```python
from build123d import *

# Parameters (mm, degrees)
SKETCH_1_W          = 15
SKETCH_1_H          = 5
EXTRUDE_1_DEPTH     = 10
SKETCH_2_W          = 15
SKETCH_2_H          = 15
EXTRUDE_2_DEPTH     = 5
SKETCH_3_R          = 1.25
CUT_EXTRUDE_1_DEPTH = 6
SKETCH_4_R          = 1.25
CUT_EXTRUDE_2_DEPTH = 5


with BuildPart() as part:
    # 草图1 → 凸台-拉伸1 (new body)
    with BuildSketch(Plane(origin=(0, 0, 0), x_dir=(1, 0, 0), z_dir=(0, 1, 0))):
        with Locations((7.5, 2.5)):
            Rectangle(SKETCH_1_W, SKETCH_1_H)
    extrude(amount=EXTRUDE_1_DEPTH)

    # 草图2 → 凸台-拉伸2 (add)
    with BuildSketch(Plane(origin=(0, 10, 0), x_dir=(1, 0, 0), z_dir=(0, 1, 0))):
        with Locations((7.5, -2.5)):
            Rectangle(SKETCH_2_W, SKETCH_2_H)
    extrude(amount=EXTRUDE_2_DEPTH)

    # 草图3 → 切除-拉伸1 (cut, through all)
    with BuildSketch(Plane.XY):
        with Locations((7.5, 5)):
            Circle(SKETCH_3_R)
    extrude(amount=-CUT_EXTRUDE_1_DEPTH, mode=Mode.SUBTRACT)

    # 草图4 → 切除-拉伸2 (cut)
    with BuildSketch(Plane(origin=(0, 15, 0), x_dir=(1, 0, 0), z_dir=(0, 1, 0))):
        with Locations((3, -5)):
            Circle(SKETCH_4_R)
        with Locations((12, -5)):
            Circle(SKETCH_4_R)
    extrude(amount=-CUT_EXTRUDE_2_DEPTH, mode=Mode.SUBTRACT)


solid = part.part
```
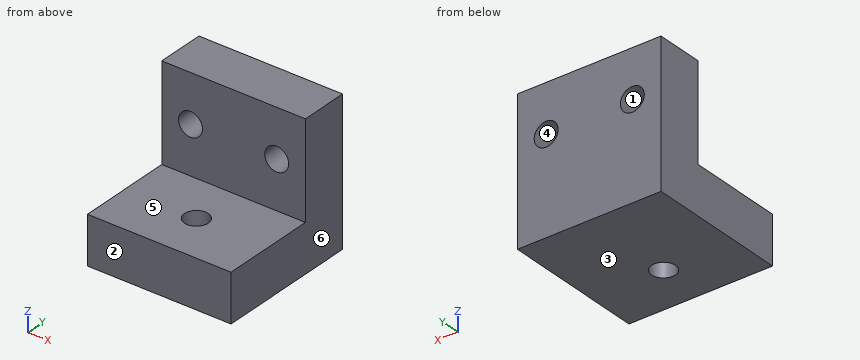
Model file for the job. Use its own axes, mm. Face numbers are marked on the shaded views. A direction names the side the tool comes from. Coordinates: 2 decimals unless noted, no trailing zeros. Write each loop counter-clockwise with the first axis right and the second up, starting at its lowest first coordinate (ties: lowest second). Pieces come first, ordered by that corner, then holes. Notation, with made-up numbers: (-20, 75.25) - (34, 75.25) arc R9 ccw to (34, 91.25) - close; hole circle Ø6 at (88.5, 77). An arc over 180 degrees is marked (long way). One line per question, with ' | ' between items. Start each with the question number.
Q1. 3-axis set-ups, long thin cutter, end or side, ignore diameter. For the marked faces 5 and 6: which of +Z, -Z, +X, -X, +Y, -Y reach the whole face in a straight line?
Q2. Cut at D-D, the plane y = 13.25. List the corners of the cut face in (x, z).
Q3. Cut at C-C, the plane z = 5. List the corners of the cut face in (x, y).
Q4. Cut at A-A, the plane x = 6.5. List the corners of the cut face in (y, z).
Q5. Pin check, flat tips, straight feed: pin 1 (5 mm diameter, centred on x = 11, z = 4.5, fed in from -Y); pin 2 (1.5 mm diameter, centred on x = 12, z = 5, fed in from +Y); pin 3 (1 mm diameter, centred on x = 6.5, y = 9, fed in from +Z). Stop position of each tip, or through.
Q6. Drill centre lines: line 1 (X direction, y = 12.2, z = 5); line 2 (Y direction, x = 7.5, z = -3.8); line 3 (Z direction, x = 3, y = 11.45). Where is each one in solid material? Low to high. Write a range as [from, to].
Q7. Pull direction Z, two halves, no side cores. Call the marked faces 1, 2, 3 and 4: pulls with the +Z half, pulls with the -Z half, needs draft (parallel to the pull), parting line crosses it, or undercut.
Q8. Cut at B-B, the plane y = 5. List the corners of the cut face in (x, z).
Answer below:
1) face 5: +Z, +X, -X, -Y | face 6: +Z, -Z, +X, +Y, -Y
2) outline: (0, -5) - (15, -5) - (15, 10) - (0, 10) - close; hole circle Ø2.5 at (3, 5); hole circle Ø2.5 at (12, 5)
3) outline: (0, 10) - (1.75, 10) - (1.75, 15) - (0, 15) - close; (4.25, 10) - (10.75, 10) - (10.75, 15) - (4.25, 15) - close; (13.25, 10) - (15, 10) - (15, 15) - (13.25, 15) - close
4) outline: (0, -5) - (4.25, -5) - (4.25, 0) - (0, 0) - close; (5.75, -5) - (15, -5) - (15, 10) - (10, 10) - (10, 0) - (5.75, 0) - close
5) pin 1: y = 10 | pin 2: through | pin 3: z = 0
6) line 1: [0, 1.75], [4.25, 10.75], [13.25, 15] | line 2: [0, 3.75], [6.25, 15] | line 3: [-5, 3.75], [6.25, 10]
7) face 1: undercut | face 2: needs draft | face 3: pulls with the -Z half | face 4: undercut
8) outline: (0, -5) - (6.25, -5) - (6.25, 0) - (0, 0) - close; (8.75, -5) - (15, -5) - (15, 0) - (8.75, 0) - close
